from build123d import *

# Parameters (mm, degrees)
SALIENTE_EXTRUIR1_DEPTH = 5
CROQUIS2_R              = 11
CROQUIS2_R_2            = 6.5
CROQUIS2_R_3            = 2
CORTAR_EXTRUIR4_DEPTH   = 220


with BuildPart() as part:
    # Croquis1 → Saliente-Extruir1 (new body)
    with BuildSketch(Plane.XY):
        with BuildLine():
            Line((120, 0), (370, 0))
            ThreePointArc((370, 0), (400, 30), (370, 60))
            Line((370, 60), (120, 60))
            ThreePointArc((120, 60), (90, 30), (120, 0))
        make_face()
    extrude(amount=SALIENTE_EXTRUIR1_DEPTH)

    # Croquis2 → Cortar-Extruir4 (cut)
    with BuildSketch(Plane.XY.offset(5)):
        with Locations((370, 30)):
            Circle(CROQUIS2_R)
        with Locations((150, 30)):
            Circle(CROQUIS2_R_2)
        with Locations((120, 30)):
            Circle(CROQUIS2_R_3)
        with Locations((120, 22)):
            Circle(CROQUIS2_R_3)
        with Locations((120, 38)):
            Circle(CROQUIS2_R_3)
        with Locations((112, 30)):
            Circle(CROQUIS2_R_3)
    extrude(amount=-CORTAR_EXTRUIR4_DEPTH, mode=Mode.SUBTRACT)


solid = part.part
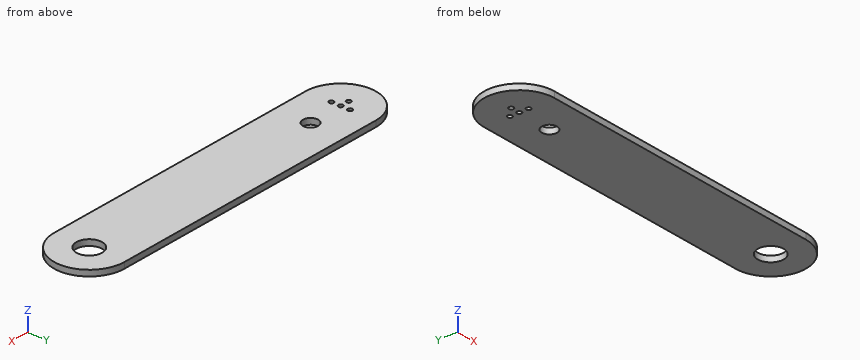
The listing builds one solid part. Answer for the finished solid, in the listing's coordinates (mm). Give positions to 0.01 mm unless a question says otherwise; leave off trailing zeros. Loops run counter-clockwise (first coordinate to the right, second up) from the corner with the lowest first, then second, coordinate; pieces in that order, holes last. Notation, with made-up numbers: (84.5, 45.5) - (130.5, 45.5) arc R29 cw to (130.5, 73.5) - close; hole circle Ø4 at (86.5, 29). An arc over 180 degrees is marked (long way). Use one line per item in the form item = value.
1. Given pin 1 Ø2.5 at (x, y) = (120, 38) entering from -Z, flat-ended and moving along its own axis, determine where the tip first touches the part or whether it passes through.
Calculated:
pin_1 = through
2. Section A-A on z = 2 is taken. Give the vertices of the cut face in (x, y), then the cut area to 3 significant figures.
Calculated:
outline = (120, 0) - (370, 0) arc R30 ccw to (370, 60) - (120, 60) arc R30 ccw to start; hole circle Ø4 at (112, 30); hole circle Ø4 at (120, 22); hole circle Ø4 at (120, 30); hole circle Ø4 at (120, 38); hole circle Ø13 at (150, 30); hole circle Ø22 at (370, 30)
area = 17,300 mm^2
3. Find the intervals of material crossed by line 1 along Y through (x, z) = (150, 1); line 2 along Y through (x, z) = (120, 3.05); line 3 along Y through (x, z) = (112, 2.75), in increasing order. Write a range as [from, to].
Calculated:
line_1 = [0, 23.5], [36.5, 60]
line_2 = [0, 20], [24, 28], [32, 36], [40, 60]
line_3 = [1.09, 28], [32, 58.91]
